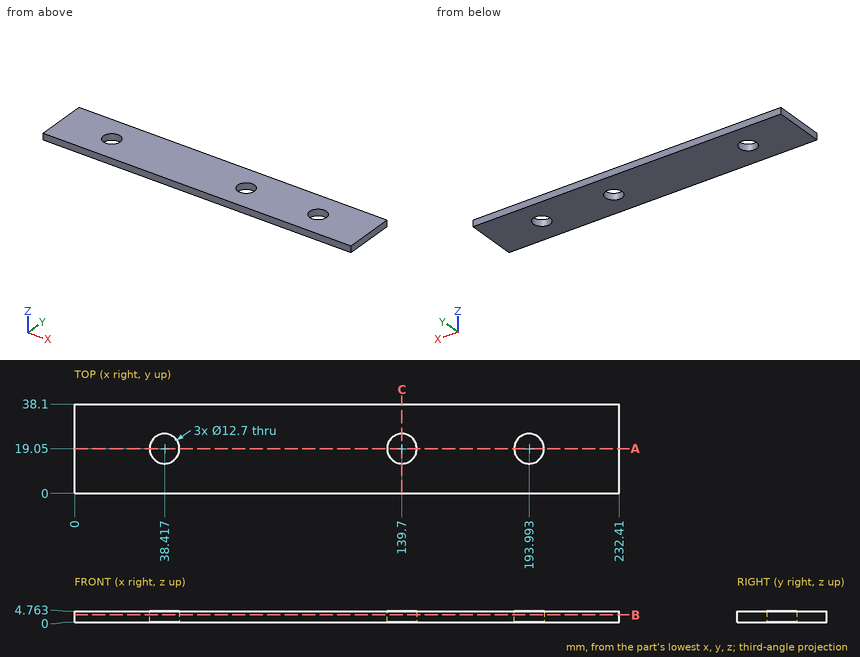
Design review of the part shown in the three views and the two pictorial views. Dimensions are in mm from the part's minimum x, y and z. Round coordinates to 2 decimals unless told otherwise and drop trailing zeros. Write each loop counter-clockwise with the first axis right and the second up, starting at its lowest first coordinate (ties: lowest second). Pieces come first, ordered by that corner, then holes. Notation, with made-up numbers: M 22.5,24 L 77.5,24 A11 cw 77.5,31 Z; hole C -5,2.25 d10. An arc over 180 degrees is marked long. Use a Markdown table: item, result. Add a question column.
Q1. We need section C-C, the plane x = 139.7. State the section outline as (y, z) points.
Q2. We need section A-A, the plane y = 19.05. State the section outline as (x, z) points.
Q3. To check wall thickness, follow line 1 (X direction, y = 19.05, z = 3.65); line 2 (X direction, y = 19.5, z = 1.4) (1 decimal); line 3 (Y direction, x = 199, z = 2.2) (1 decimal). State the ranges of each line that lie inside material, in increasing order.
Q4. We need section B-B, the plane z = 3.25. State the section outline as (x, y) points.
Findings below:
| question | item | result |
|---|---|---|
| 1 | outline | M 0,0 L 12.7,0 L 12.7,4.76 L 0,4.76 Z; M 25.4,0 L 38.1,0 L 38.1,4.76 L 25.4,4.76 Z |
| 2 | outline | M 0,0 L 32.07,0 L 32.07,4.76 L 0,4.76 Z; M 44.77,0 L 133.35,0 L 133.35,4.76 L 44.77,4.76 Z; M 146.05,0 L 187.64,0 L 187.64,4.76 L 146.05,4.76 Z; M 200.34,0 L 232.41,0 L 232.41,4.76 L 200.34,4.76 Z |
| 3 | line 1 | x = 0 to 32.07, 44.77 to 133.35, 146.05 to 187.64, 200.34 to 232.41 |
| 3 | line 2 | x = 0 to 32.1, 44.8 to 133.4, 146 to 187.7, 200.3 to 232.4 |
| 3 | line 3 | y = 0 to 15.1, 23 to 38.1 |
| 4 | outline | M 0,0 L 232.41,0 L 232.41,38.1 L 0,38.1 Z; hole C 38.42,19.05 d12.7; hole C 139.7,19.05 d12.7; hole C 193.99,19.05 d12.7 |
